from build123d import *

# Parameters (mm, degrees)
F2_R     = 5
F3_DEPTH = 30
F5_DEPTH = 25


with BuildPart() as f1:
    # F0 (on Front) → F1 (revolve)
    with BuildSketch(Plane.XZ):
        Polygon((-22.083245, 12.95), (-22.083245, 0), (3.116755, 0), (3.116755, 12.95), (0.016755, 12.95), (0.016755, 7.95), (-18.983245, 7.95), (-18.983245, 12.95), align=None)
    revolve(axis=Axis((-7.986653, 0, 0), (-1, 0, 0)))

    # F2 (on face) → F3 (cut)
    with BuildSketch(Plane.YZ.offset(3.116755)):
        Circle(F2_R)
    extrude(amount=-F3_DEPTH, mode=Mode.SUBTRACT)

    # F4 (on Right) → F5 (join)
    with BuildSketch(Plane.YZ):
        Polygon((-37.379272, 29.986372), (-46.934061, 29.986372), (-46.934061, -8.687175), (9.331752, -8.687175), (9.331752, 29.986372), (-23.615412, 29.986372), (-23.615412, 5.463502), (-37.379272, 5.463502), align=None)
    extrude(amount=F5_DEPTH)


solid = f1.part
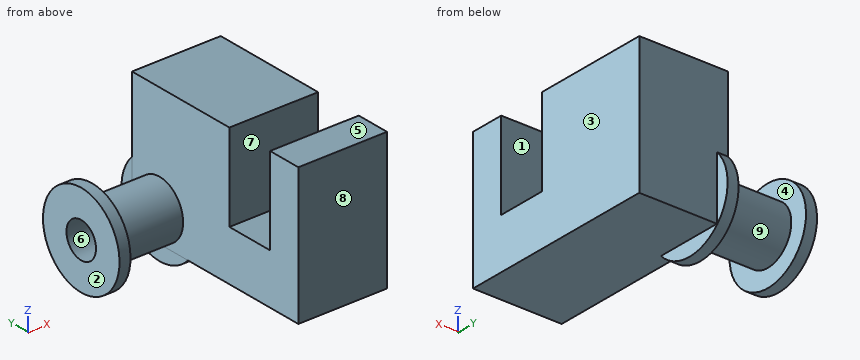
For this review, take the finished solid that the model builds, in its own axes (mm). Face numbers are marked on the shaded views. A direction names the side the tool comes from. Round coordinates to 2 decimals unless told otherwise and drop trailing zeros. Order: outer loops, then holes, each group sorted by start corner. A loop starts at its lowest first (then second) coordinate and runs counter-clockwise, first axis right, second up. Notation, with made-up numbers: M -13,8 L -8,8 A14 ccw -8,19 Z; hole C 78,67 d2. An arc over 180 degrees is marked long. Write each question's results on one line, items separated by ' | '. Start each with the question number.
1. To check wall thickness, follow L1, parallel to Y at x = 23, z = 7; L2, parallel to X at y = 8, z = -5; L3, parallel to X at y = -18.5, z = -8.5. State the ranges of each line that lie inside material, in increasing order. Write a range as [from, to].
2. Clearance check with flat-ended pins moving along their axes: pin 1 Ø11.5 at (y, z) = (-26, 5.5) entering from -X; pin 2 Ø12.5 at (x, y) = (16, -24) entering from -Z; pin 3 Ø7.5 at (x, z) = (9.5, 10) entering from +Y. State where each tip first meets the part, or that it passes through.
3. Add section D-D (x = -18). State the section outline as (y, z) points.
4. Add section B-B (x = 2). State the section outline as (y, z) points.
5. Draft analysis for pull direction X (two halves, no side actions). For the marked faces 1, 2, 3 and 4, state which applies: pulls with the +X half, pulls with the -X half, needs draft (parallel to the pull), parting line crosses it, or undercut.
6. Tool access review of the marked faces 5, 6, 7, 8 and 9: name each direction out of +Z, -Z, +X, -X, +Y, -Y from which nothing blocks a thin tool from reaching the whole face with its end or side.
Output values:
1) L1: [-46.93, -37.38], [-23.62, 9.33] | L2: [-22.08, -18.98], [0, 25] | L3: [0, 25]
2) pin 1: x = 0 | pin 2: z = -8.69 | pin 3: y = 9.33
3) outline: C 0,0 d15.9; hole C 0,0 d10
4) outline: M -46.93,-8.69 L -9.6,-8.69 A12.95 ccw long 9.33,8.98 L 9.33,29.99 L -23.62,29.99 L -23.62,5.46 L -37.38,5.46 L -37.38,29.99 L -46.93,29.99 Z
5) face 1: needs draft | face 2: pulls with the -X half | face 3: pulls with the +X half | face 4: undercut
6) face 5: +Z, +X, -X, +Y, -Y | face 6: -X | face 7: +Z, +X, -X | face 8: +Z, -Z, +X, -X, -Y | face 9: none
